CAD build for the part. Positions are in the model's coordinates, mm. Face numbers are marked on the shaded views. A direction names the side the tool comes from. Give positions to 0.01 mm unless a question says otherwise; leave off trailing zeros. Loops run counter-clockwise (first coordinate to the right, second up) from the corner with the lowest first, then second, coordinate; pieces in that order, holes last. Notation, with made-up numbers: (64.5, 62.25) - (102.5, 62.25) arc R29 cw to (102.5, 89.25) - close; hole circle Ø8 at (27.25, 58.25). An arc over 180 degrees is marked (long way). Return JSON: item names as keys, results as strings.
from build123d import *

# Parameters (mm, degrees)
SKETCH_1_W      = 400
SKETCH_1_H      = 400
EXTRUDE_1_DEPTH = 50
SKETCH_2_W      = 50
SKETCH_2_H      = 50
EXTRUDE_2_DEPTH = 400
SKETCH_3_W      = 50
SKETCH_3_H      = 50
EXTRUDE_3_DEPTH = 400
SKETCH_4_W      = 50
SKETCH_4_H      = 50
EXTRUDE_4_DEPTH = 400
SKETCH_5_W      = 50
SKETCH_5_H      = 50
EXTRUDE_5_DEPTH = 400
SKETCH_6_W      = 400
SKETCH_6_H      = 400
EXTRUDE_6_DEPTH = 50
SKETCH_7_W      = 400
SKETCH_7_H      = 50
EXTRUDE_7_DEPTH = 400


with BuildPart() as part:
    # 草图1 → 凸台-拉伸1 (new body)
    with BuildSketch(Plane.XY):
        Rectangle(SKETCH_1_W, SKETCH_1_H)
    extrude(amount=EXTRUDE_1_DEPTH)

    # 草图2 → 凸台-拉伸2 (add)
    with BuildSketch(Plane.XY):
        with Locations((175, 175)):
            Rectangle(SKETCH_2_W, SKETCH_2_H)
    extrude(amount=EXTRUDE_2_DEPTH)

    # 草图3 → 凸台-拉伸3 (add)
    with BuildSketch(Plane.XY):
        with Locations((-175, 175)):
            Rectangle(SKETCH_3_W, SKETCH_3_H)
    extrude(amount=EXTRUDE_3_DEPTH)

    # 草图4 → 凸台-拉伸4 (add)
    with BuildSketch(Plane.XY):
        with Locations((175, -175)):
            Rectangle(SKETCH_4_W, SKETCH_4_H)
    extrude(amount=EXTRUDE_4_DEPTH)

    # 草图5 → 凸台-拉伸5 (add)
    with BuildSketch(Plane.XY):
        with Locations((-175, -175)):
            Rectangle(SKETCH_5_W, SKETCH_5_H)
    extrude(amount=EXTRUDE_5_DEPTH)

    # 草图6 → 凸台-拉伸6 (add)
    with BuildSketch(Plane.XY):
        Rectangle(SKETCH_6_W, SKETCH_6_H)
    extrude(amount=EXTRUDE_6_DEPTH)

    # 草图7 → 凸台-拉伸7 (add)
    with BuildSketch(Plane(origin=(0, 200, 0), x_dir=(1, 0, 0), z_dir=(0, 1, 0))):
        Rectangle(SKETCH_7_W, SKETCH_7_H)
    extrude(amount=EXTRUDE_7_DEPTH)


solid = part.part
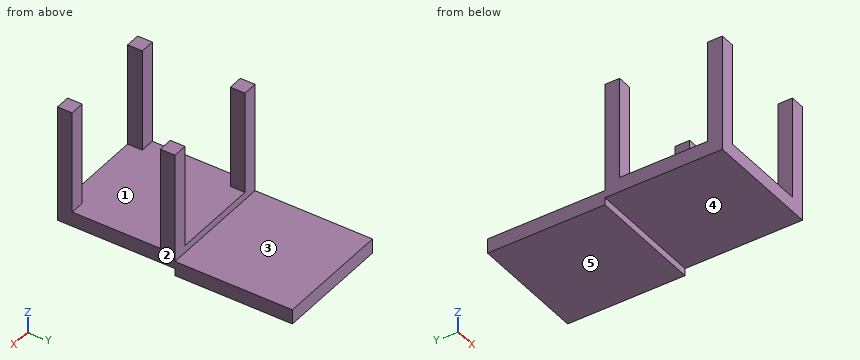
1. Cut at B-B, the plane x = 94.5. Write the cut outline in (y, z).
Values follow:
{"outline": "(-200, 0) - (200, 0) - (200, -25) - (600, -25) - (600, 25) - (200, 25) - (200, 50) - (-200, 50) - close"}
2. Drill centre lines: probe 1 along Y at (x, z) = (-157, 371); probe 2 along Z at (x, y) = (47.5, 76). Where is each one in solid material? Low to high.
Values follow:
{"probe 1": "y = -200 to -150, 150 to 200", "probe 2": "z = 0 to 50"}
3. Cut at A-A, the plane z = 198. Write the cut outline in (x, y).
Values follow:
{"outline": "(-200, -200) - (-150, -200) - (-150, -150) - (-200, -150) - close; (-200, 150) - (-150, 150) - (-150, 200) - (-200, 200) - close; (150, -200) - (200, -200) - (200, -150) - (150, -150) - close; (150, 150) - (200, 150) - (200, 200) - (150, 200) - close"}
4. Which spindle directions (+Z, -Z, +X, -X, +Y, -Y) get a long thin tool onto all of the face, cutting with end or side? Do the marked faces 3, 4 and 5. Say none if no direction does.
Values follow:
{"face 3": "+Z, +X, -X, +Y", "face 4": "-Z, +X, -X, -Y", "face 5": "-Z, +X, -X, +Y, -Y"}
5. Cut at C-C, the plane y = 339. Write the cut outline in (x, z).
Values follow:
{"outline": "(-200, -25) - (200, -25) - (200, 25) - (-200, 25) - close"}
6. Drop flat-ended pins along their axis: P1, Ø7.5, axis at x = -61.5, z = -16, coming from the -Y side; P2, Ø8, axis at x = -143.5, y = 177, coming from the -Z side. Give the stop position or say it passes through.
Values follow:
{"P1": "stops at y = 200", "P2": "stops at z = 0"}
7. Pull direction Y, two halves, no side cores. Call the marked faces 1 and 2: +Y half, -Y half, draft (parallel to the pull), parting line (faces both ways), or undercut.
Values follow:
{"face 1": "undercut", "face 2": "draft"}
